```python
from build123d import *

# Parameters (mm, degrees)
F0_W     = 82.296
F0_H     = 153.416
F1_DEPTH = 16.256
F2_W     = 72.136
F2_H     = 143.256
F3_DEPTH = 7.62
F4_R     = 5.08
F5_R     = 5.08
F6_R     = 5.08
F7_R     = 5.08
F8_R     = 3.81
F9_R     = 3.81


with BuildPart() as f1:
    # F0 (on Front) → F1 (new body)
    with BuildSketch(Plane.XZ):
        Rectangle(F0_W, F0_H)
    extrude(amount=F1_DEPTH)

    # F2 (on face) → F3 (cut)
    with BuildSketch(Plane.XZ.offset(16.256)):
        Rectangle(F2_W, F2_H)
    extrude(amount=-F3_DEPTH, mode=Mode.SUBTRACT)

    # F4
    f4_edges = [f1.edges().sort_by_distance(p)[0] for p in [
        (-36.068, -12.446, 71.628),
    ]]
    fillet(f4_edges, radius=F4_R)

    # F5
    f5_edges = [f1.edges().sort_by_distance(p)[0] for p in [
        (36.068, -12.446, 71.628),
    ]]
    fillet(f5_edges, radius=F5_R)

    # F6
    f6_edges = [f1.edges().sort_by_distance(p)[0] for p in [
        (36.068, -12.446, -71.628),
    ]]
    fillet(f6_edges, radius=F6_R)

    # F7
    f7_edges = [f1.edges().sort_by_distance(p)[0] for p in [
        (-36.068, -12.446, -71.628),
    ]]
    fillet(f7_edges, radius=F7_R)

    # F8
    f8_edges = [f1.edges().sort_by_distance(p)[0] for p in [
        (41.148, -16.256, 0),
        (-41.148, -16.256, 0),
    ]]
    fillet(f8_edges, radius=F8_R)

    # F9
    f9_edges = [f1.edges().sort_by_distance(p)[0] for p in [
        (0, -16.256, 76.708),
        (0, -16.256, -76.708),
    ]]
    fillet(f9_edges, radius=F9_R)


solid = f1.part
```
The listing builds one solid part. Answer for the finished solid, in the listing's coordinates (mm). A direction names the side the tool comes from. Round coordinates to 2 decimals unless told otherwise and drop trailing zeros. Order: outer loops, then holes, each group sorted by start corner. A loop starts at its lowest first (then second) coordinate and runs counter-clockwise, first axis right, second up. Notation, with made-up numbers: (24, 72.25) -> (32, 72.25) arc R25 ccw to (32, 84.25) -> close; hole circle Ø10 at (-15.5, 73.25). An arc over 180 degrees is marked (long way). Answer as CSV lines item,"result". Start each with the question number.
(1) The part is cut by section C-C (z = 30.5). Determine the outline of the cut face in (x, y), then the cut area to 3 significant figures.
(2) The part is cut by section A-A (y = -10.25). Determine the outline of the cut face in (x, z).
(3) A tool of negligible diameter and unlimited length cuts with its end or side. For faces 1 (the face through (34.54, -12.39, 70.18)), 2 (the face through (-40.062, -6.31, -75.562)), from which of +Z, -Z, +X, -X, +Y, -Y can it reach the whole face along a straight path? Write none if from no direction.
(4) Flat-ended cylindrical pins translate along their axes: pin 1 Ø2.5 at (y, z) = (-14, 18.5) entering from +X; pin 2 Ø6 at (x, z) = (2.5, 28.5) entering from -Y. Find the tip coordinate at first contact, or state that the pin passes through.
(5) The part is cut by section B-B (x = 21). Determine the outline of the cut face in (y, z), then the cut area to 3 significant figures.
(6) Find the intervals of material crossed by probe 1 along X at (y, z) = (-11.25, -51.5); probe 2 along Z at (x, y) = (-24.5, -10.75); probe 3 along Y at (x, z) = (8, -42), in increasing order. Write a range as from..to.
(7) For a pull along X with two mould halves and no side action, classify faces 3 (the face through (40, -15.17, 1.02)), 4 (the face through (-1, -6, -76.708)), 5 (the face through (-34.54, -12.39, 70.18)) as +X half, -X half, draft (parallel to the pull), parting line (faces both ways), or undercut.
Evaluation:
1,outline,"(-41.15, -12.45) arc R3.81 ccw to (-37.34, -16.26) -> (-36.07, -16.26) -> (-36.07, -8.64) -> (36.07, -8.64) -> (36.07, -16.26) -> (37.34, -16.26) arc R3.81 ccw to (41.15, -12.45) -> (41.15, 0) -> (-41.15, 0) -> close"
1,area,"782 mm²"
2,outline,"(-41.15, -72.9) arc R3.81 ccw to (-37.34, -76.71) -> (37.34, -76.71) arc R3.81 ccw to (41.15, -72.9) -> (41.15, 72.9) arc R3.81 ccw to (37.34, 76.71) -> (-37.34, 76.71) arc R3.81 ccw to (-41.15, 72.9) -> close; hole (-36.07, -66.55) arc R5.08 ccw to (-30.99, -71.63) -> (30.99, -71.63) arc R5.08 ccw to (36.07, -66.55) -> (36.07, 66.55) arc R5.08 ccw to (30.99, 71.63) -> (-30.99, 71.63) arc R5.08 ccw to (-36.07, 66.55) -> close"
3,face 1,"-Y"
3,face 2,"-Z, -X, +Y, -Y"
4,pin 1,"x = 41.14"
4,pin 2,"y = -8.64"
5,outline,"(-16.26, -72.9) arc R3.81 ccw to (-12.45, -76.71) -> (0, -76.71) -> (0, 76.71) -> (-12.45, 76.71) arc R3.81 ccw to (-16.26, 72.9) -> (-16.26, 71.63) -> (-8.64, 71.63) -> (-8.64, -71.63) -> (-16.26, -71.63) -> close"
5,area,"1,400 mm²"
6,probe 1,"-41.15..-36.07, 36.07..41.15"
6,probe 2,"-76.71..-71.63, 71.63..76.71"
6,probe 3,"-8.64..0"
7,face 3,"+X half"
7,face 4,"draft"
7,face 5,"undercut"
